Part model, mm, in its own coordinate system. Face numbers are marked on the shaded views. A direction names the side the tool comes from. Round coordinates to 2 decimals unless told otherwise and drop trailing zeros. Order: outer loops, then holes, each group sorted by start corner. A loop starts at its lowest first (then second) coordinate and runs counter-clockwise, first axis right, second up. Notation, with made-up numbers: (34, 86.5) -> (72, 86.5) arc R12 ccw to (72, 94.5) -> close; hole circle Ø8 at (30, 56.5). An arc over 180 degrees is marked (long way). Use CSV: the item, a comma, the result in double quotes.
```python
from build123d import *

# Parameters (mm, degrees)
F0_R     = 11
F0_R_2   = 4
F1_DEPTH = 7
F2_R     = 9.55
F2_R_2   = 6.2
F3_DEPTH = 0.5
F4_R     = 9.55
F4_R_2   = 6.2
F5_DEPTH = 0.5
F6_R     = 0.3
F7_R     = 0.3
F8_R     = 0.3


with BuildPart() as f1:
    # F0 (on Front) → F1 (new body)
    with BuildSketch(Plane.XZ):
        Circle(F0_R)
        Circle(F0_R_2, mode=Mode.SUBTRACT)
    extrude(amount=F1_DEPTH)

    # F2 (on face) → F3 (cut)
    with BuildSketch(Plane(origin=(0, 0, 0), x_dir=(-1, 0, 0), z_dir=(0, 1, 0))):
        Circle(F2_R)
        Circle(F2_R_2, mode=Mode.SUBTRACT)
    extrude(amount=-F3_DEPTH, mode=Mode.SUBTRACT)

    # F4 (on face) → F5 (cut)
    with BuildSketch(Plane.XZ.offset(7)):
        Circle(F4_R)
        Circle(F4_R_2, mode=Mode.SUBTRACT)
    extrude(amount=-F5_DEPTH, mode=Mode.SUBTRACT)

    # F6
    f6_edges = [f1.edges().sort_by_distance(p)[0] for p in [
        (-11, 0, 0),
    ]]
    fillet(f6_edges, radius=F6_R)

    # F7
    f7_edges = [f1.edges().sort_by_distance(p)[0] for p in [
        (-11, -7, 0),
        (-4, -7, 0),
    ]]
    fillet(f7_edges, radius=F7_R)

    # F8
    f8_edges = [f1.edges().sort_by_distance(p)[0] for p in [
        (-4, 0, 0),
    ]]
    fillet(f8_edges, radius=F8_R)


solid = f1.part
```
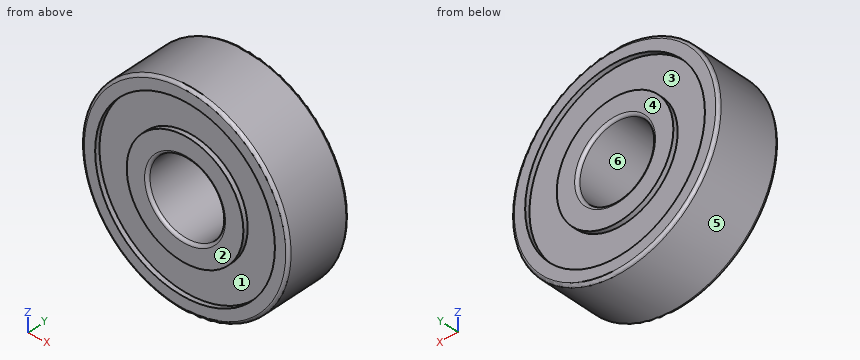
(1) Which spindle directions (+Z, -Z, +X, -X, +Y, -Y) get a long thin tool onto all of the face, cutting with end or side? Do the marked faces 1, 2 and 3. Say none if no direction does.
Reply:
face 1,"-Y"
face 2,"+Z, -Z, +X, -X, -Y"
face 3,"+Y"
(2) Drop flat-ended pins along their axis: P1, Ø1.5, axis at y = -1.5, z = -2.5, coming from the +X side; P2, Ø4, axis at x = -7, y = -5, coming from the +Z side; P3, Ø1, axis at x = -6, y = -3.5, coming from the +Z side. Give the stop position or say it passes through.
Reply:
P1,"x = 10.86"
P2,"z = 9.8"
P3,"z = 9.53"
(3) Pull direction Z, two halves, no side cores. Call the marked faces 4, 5 and 6: released by +Z, released by -Z, zero draft, split by the parting line, or undercut.
Reply:
face 4,"zero draft"
face 5,"split by the parting line"
face 6,"undercut"
(4) Probe probe 1 along Z at (x, y) = (0, -3.25); probe 2 along Z at (x, y) = (0, -6.7); probe 3 along Z at (x, y) = (0, -6.9). List the from-to ranges inside material, lowest first. Write a range as [from, to].
Reply:
probe 1,"[-11, -4], [4, 11]"
probe 2,"[-11, -9.55], [-6.2, -4], [4, 6.2], [9.55, 11]"
probe 3,"[-10.92, -9.55], [-6.2, -4.08], [4.08, 6.2], [9.55, 10.92]"
(5) Cut at C-C, the plane y = -2.5. Give the cut face in (x, z), then the cut area to 3 significant figures.
Reply:
outline,"circle Ø22 at (0, 0); hole circle Ø8 at (0, 0)"
area,"330 mm2"
